CAD build for the part. Positions are in the model's coordinates, mm. A direction names the side the tool comes from. Give positions to 0.01 mm unless a question says otherwise; leave off trailing zeros. Order: outer loops, then holes, each group sorted by start corner. A loop starts at its lowest first (then second) coordinate and runs counter-clockwise, first axis right, second up.
Item 1: Band-saw the part on D-D on x = -20. Give the cut face in (y, z), plus the area to 3 significant figures.
Item 2: Wall check: L1, parallel to X at y = 0.65, z = 0; L2, parallel to Z at x = 0, y = 16.5; L3, parallel to Z at x = 25, y = 5.5. Give the ranges that are in metal, low to high.
Item 3: Band-saw the part on A-A on x = 0. Give the cut face in (y, z), plus the area to 3 significant figures.
Item 4: Band-saw the part on B-B on z = 20. Give the cut face in (x, y).
Item 5: Band-saw the part on C-C on y = 3.25. Give the cut face in (x, z).
Item 6: Flat gauge pins, fed straight in: P1, Ø8, axis at y = 26.5, z = -17, coming from the +X side; P2, Ø3.5, axis at x = 0, z = -20, coming from the +Y side; P3, Ø2.5, axis at x = -30, z = -0.5, coming from the +Y side; P4, Ø2.5, axis at x = 0, z = 20, coming from the -Y side. Where does each tip first touch, or does it go through?
Item 7: Two-plate mould, pull along X, no slides. Class faces 3 (the flat face through (0.2, 30, 30.2)), 4 (the cylindrical face through (-18.463, 0.493, 0.202)), 5 (the cylindrical face through (-30.565, 24.93, 3.505)), 6 (the cylindrical face through (31.232, 14.79, -4.101)): released by +X, released by -X, zero draft, split by the parting line, or undercut.
Item 8: Which spindle directions (+Z, -Z, +X, -X, +Y, -Y) get a long thin tool onto all of the face, cutting with end or side? Do faces 1 (the cylindrical face through (-0.594, 0.493, 18.568)), 2 (the flat face through (0, 1, 0)). Say none if no direction does.
```python
from build123d import *

# Parameters (mm, degrees)
SKETCH1_R           = 31.5
BOSS_EXTRUDE2_DEPTH = 30
SKETCH2_R           = 30
CUT_EXTRUDE1_DEPTH  = 29
SKETCH3_R           = 1.55
CUT_EXTRUDE2_DEPTH  = 54.70754137
CUT_EXTRUDE3_START  = 20
CUT_EXTRUDE3_DEPTH  = 10


# Read off the part's stored shape, not the designer's step: Cut-Extrude3
with BuildPart() as part:
    # Sketch1 → Boss-Extrude2 (new body)
    with BuildSketch(Plane(origin=(0, 0, 0), x_dir=(1, 0, 0), z_dir=(0, 1, 0))):
        with Locations(Location((0, 0, 0), (0, 0, 270))):
            Circle(SKETCH1_R)
    extrude(amount=BOSS_EXTRUDE2_DEPTH)

    # Sketch2 → Cut-Extrude1 (cut)
    with BuildSketch(Plane(origin=(0, 30, 0), x_dir=(1, 0, 0), z_dir=(0, 1, 0))):
        with Locations(Location((0, 0, 0), (0, 0, 270))):
            Circle(SKETCH2_R)
    extrude(amount=-CUT_EXTRUDE1_DEPTH, mode=Mode.SUBTRACT)

    # Sketch3 → Cut-Extrude2 (cut, through all)
    with BuildSketch(Plane.XZ):
        with Locations(Location((0, 20, 0), (0, 0, 270))):
            Circle(SKETCH3_R)
        with Locations(Location((-20, 0, 0), (0, 0, 270))):
            Circle(SKETCH3_R)
        with Locations(Location((0, -20, 0), (0, 0, 270))):
            Circle(SKETCH3_R)
        with Locations(Location((20, 0, 0), (0, 0, 270))):
            Circle(SKETCH3_R)
    extrude(amount=-CUT_EXTRUDE2_DEPTH, mode=Mode.SUBTRACT)

    # Cut-Extrude3 outline → Cut-Extrude3 (cut)
    with BuildSketch(Plane(origin=(0, 0, 0), x_dir=(1, 0, 0), z_dir=(0, 1, 0)).offset(CUT_EXTRUDE3_START)):
        with BuildLine():
            ThreePointArc((-29.299835483, 6.443573593), (-30.039033671, 6.596315408), (-30.792713244, 6.637681152))
            ThreePointArc((-30.792713244, 6.637681152), (-31.45908722, 1.604939654), (-31.308347945, -3.469488288))
            ThreePointArc((-31.308347945, -3.469488288), (-30.554371668, -3.505038211), (-29.803467005, -3.428316566))
            ThreePointArc((-29.803467005, -3.428316566), (-29.961035448, 1.528513956), (-29.299835483, 6.443573593))
        make_face()
    extrude(amount=CUT_EXTRUDE3_DEPTH, mode=Mode.SUBTRACT)


solid = part.part
```
The answers:
1. outline: (0, -24.34) - (30, -24.34) - (30, -22.36) - (1, -22.36) - (1, -1.55) - (0, -1.55) - close; (0, 1.55) - (1, 1.55) - (1, 22.36) - (30, 22.36) - (30, 24.34) - (0, 24.34) - close
1. area: 160 mm2
2. L1: x = -31.5 to -21.55, -18.45 to 18.45, 21.55 to 31.5
2. L2: z = -31.5 to -30, 30 to 31.5
2. L3: z = -19.16 to -16.58, 16.58 to 19.16
3. outline: (0, -31.5) - (30, -31.5) - (30, -30) - (1, -30) - (1, -21.55) - (0, -21.55) - close; (0, -18.45) - (1, -18.45) - (1, 18.45) - (0, 18.45) - close; (0, 21.55) - (1, 21.55) - (1, 30) - (30, 30) - (30, 31.5) - (0, 31.5) - close
3. area: 144 mm2
4. outline: (-24.34, 0) - (-1.55, 0) - (-1.55, 1) - (-22.36, 1) - (-22.36, 30) - (-24.34, 30) - close; (1.55, 0) - (24.34, 0) - (24.34, 30) - (22.36, 30) - (22.36, 1) - (1.55, 1) - close
5. outline: circle Ø63 at (0, 0); hole circle Ø60 at (0, 0)
6. P1: stops at x = 28.69
6. P2: stops at y = 1
6. P3: stops at y = 20
6. P4: passes through
7. face 3: zero draft
7. face 4: undercut
7. face 5: undercut
7. face 6: split by the parting line
8. face 1: +Y, -Y
8. face 2: +Y
